```python
from build123d import *

# Parameters (mm, degrees)
F1_DEPTH = 5.75


# Not quite as in the source:
# - ends of sketch curves that miss each other by under 0.0002 mm in the source are joined


with BuildPart() as f1:
    # F0 (on Top) → F1 (new body)
    with BuildSketch(Plane.XY):
        with BuildLine():
            ThreePointArc((-54.3633709611, 8.0368382821), (-55.1570277624, 7.8000823804), (-55.5, 7.046216))
            Line((-55.5, 7.046216), (-55.5, -13.228097))
            ThreePointArc((-55.5, -13.228097), (2.4981253193, -17.3024292075), (60.5000000667, -13.2818254774))
            Line((60.5000000667, -13.2818254774), (60.5, 6.993434))
            ThreePointArc((60.5, 6.993434), (60.1573766387, 7.7469961772), (59.3642880901, 7.9841823422))
            ThreePointArc((59.3642880901, 7.9841823422), (2.4986576004, 4.1208007581), (-54.3633709611, 8.0368382821))
        make_face()
    extrude(amount=F1_DEPTH)


solid = f1.part
```
Source: CAD feature listing. Evaluate the final solid. Frame: model axes, mm. Round coordinates to 2 decimals unless told otherwise and drop trailing zeros. Loops run counter-clockwise (first coordinate to the right, second up) from the corner with the lowest first, then second, coordinate; pieces in that order, holes last.
1. Section query C-C on y = -14.5. Output: boundary loops of the cut face in (x, z).
2. Ray query, L1, parallel to Y at x = 23.5, z = 3.05; L2, parallel to Y at x = -43.5, z = 2.9. Return the intervals inside material, ascending.
3. Mould query, pull axis Y, two halves, no side actions, for faces 1 (the cylindrical face through (3.3, 4.12, 2.83)), 2 (the flat face through (-55.5, -3, 3)), 3 (the cylindrical face through (1.7, -17.3, 2.8)). Classes: released by +Y, released by -Y, zero draft, split by the parting line, or undercut.
4. Contact query for a flat-ended pin moving along its axis: pin 1 (2 mm diameter, centred on x = -36, z = 1, fed in from +Y). Output: stop coordinate, or through.
5. Section query A-A on y = 5.5. Output: boundary loops of the cut face in (x, z), and give its area (3 significant figures).
6. Section query D-D on x = -46.5. Output: boundary loops of the cut face in (y, z), and give its area (3 significant figures).
7. Section query B-B on z = 3. Output: boundary loops of the cut face in (x, y), and give its area (3 significant figures).
Answers below:
1. outline: (-45.61, 0) - (50.99, 0) - (50.99, 5.75) - (-45.61, 5.75) - close
2. L1: y = -16.78 to 4.64
2. L2: y = -14.74 to 6.68
3. face 1: released by +Y
3. face 2: zero draft
3. face 3: released by -Y
4. pin 1: stops at y = 6.01
5. outline: (-55.5, 0) - (-31.22, 0) - (-31.22, 5.75) - (-55.5, 5.75) - close; (36.6, 0) - (60.5, 0) - (60.5, 5.75) - (36.6, 5.75) - close
5. area: 277 mm2
6. outline: (-14.4, 0) - (7.03, 0) - (7.03, 5.75) - (-14.4, 5.75) - close
6. area: 123 mm2
7. outline: (-55.5, -13.23) arc R417.59 ccw to (60.5, -13.28) - (60.5, 6.99) arc R1 ccw to (59.36, 7.98) arc R417.59 cw to (-54.36, 8.04) arc R1 ccw to (-55.5, 7.05) - close
7. area: 2,480 mm2
